```python
from build123d import *

# Parameters (mm, degrees)
F0_R     = 18
F1_DEPTH = 30
F2_R     = 15
F3_DEPTH = 30
F5_D     = 5.5
F6_SIZE  = 2


with BuildPart() as f1:
    # F0 (on Top) → F1 (new body)
    with BuildSketch(Plane.XY):
        Circle(F0_R)
    extrude(amount=F1_DEPTH)

    # F2 (on face) → F3 (join)
    with BuildSketch(Plane.XY.offset(30)):
        Circle(F2_R)
    extrude(amount=F3_DEPTH)

    # F5 (through all)
    with Locations(Plane(origin=(0, 0, 0), x_dir=(1, 0, 0), z_dir=(0, 0, -1))):
        with Locations((0, 0)):
            Hole(F5_D / 2)

    # F6
    f6_edges = [f1.edges().sort_by_distance(p)[0] for p in [
        (-15, 0, 60),
    ]]
    chamfer(f6_edges, length=F6_SIZE)


solid = f1.part
```
Design review of the part built by this model. Coordinates are the model's own, in mm. A direction names the side the tool comes from. Give positions to 0.01 mm unless a question says otherwise; leave off trailing zeros. Write each loop counter-clockwise with the first axis right and the second up, starting at its lowest first coordinate (ties: lowest second). Pieces come first, ordered by that corner, then holes. Notation, with made-up numbers: (17.25, 87) -> (53.25, 87) arc R32 cw to (53.25, 117) -> close; hole circle Ø8 at (-38, -29). An arc over 180 degrees is marked (long way). Answer in a Markdown table with one row per item.
(1) To check wall thickness, follow probe 1 along Y at (x, z) = (0, 38); probe 2 along Y at (x, z) = (0, 20); probe 3 along Z at (x, y) = (14, -9). State the ranges of each line that lie inside material, in increasing order.
Results:
| item | result |
|---|---|
| probe 1 | -15 to -2.75, 2.75 to 15 |
| probe 2 | -18 to -2.75, 2.75 to 18 |
| probe 3 | 0 to 30 |
(2) Clearance check with flat-ended pins moving along their axes: pin 1 (1 mm diameter, centred on x = -6.5, z = 43, fed in from +Y); pin 2 (2 mm diameter, centred on y = 9, z = 27.5, fed in from +X); pin 3 (4 mm diameter, centred on x = -10.5, z = 35.5, fed in from +Y); pin 4 (12 mm diameter, centred on y = 2, z = 26.5, fed in from +X). State where each tip first meets the part, or that it passes through.
Results:
| item | result |
|---|---|
| pin 1 | y = 13.75 |
| pin 2 | x = 16.12 |
| pin 3 | y = 12.36 |
| pin 4 | x = 18 |
(3) Mouldability with a two-part tool opening along Y and no side actions: class faces 1 (the cylindrical face through (-2.343, 17.847, 14.79)), 2 (the flat face through (-4, 15, 30)), 3 (the cylindrical face through (0.596, 2.685, 30.42)) as +Y half, -Y half, draft (parallel to the pull), parting line (faces both ways), or undercut.
Results:
| item | result |
|---|---|
| face 1 | parting line |
| face 2 | draft |
| face 3 | undercut |
(4) For faces 4 (the cylindrical face through (-14.985, 0.66, 43.804)), 5 (the flat face through (0, -4, 0)), list the 3-axis set-ups (+Z, -Z, +X, -X, +Y, -Y) from which the entire face can be reached by the end or side of a thin tool; tool diameter is ignored.
Results:
| item | result |
|---|---|
| face 4 | +Z |
| face 5 | -Z, +X, -X, +Y, -Y |
(5) Consider section A-A (x = 0). State the section outline as (y, z) points.
Results:
| item | result |
|---|---|
| outline | (-18, 0) -> (-2.75, 0) -> (-2.75, 60) -> (-13, 60) -> (-15, 58) -> (-15, 30) -> (-18, 30) -> close; (2.75, 0) -> (18, 0) -> (18, 30) -> (15, 30) -> (15, 58) -> (13, 60) -> (2.75, 60) -> close |
(6) Consider section C-C (z = 41). State the section outline as (x, y) points, then the cut area to 3 significant figures.
Results:
| item | result |
|---|---|
| outline | circle Ø30 at (0, 0); hole circle Ø5.5 at (0, 0) |
| area | 683 mm2 |
